Autodesk Fusion 360 part; units mm, degrees
sketch "Sketch1" plane through (0, 0, 0) normal (0, 0, 1) x (1, 0, 0)
  circle A0 centre (0, 0) radius 18.25
  circle A1 centre (0, 0) radius 24.5
  circle A2 centre (0, 0) radius 17.75
  circle A3 centre (0, 0) radius 16.25
  dimension "d1" = 36.5
  dimension "d2" = 49
  dimension "d7" = 35.5
  dimension "d27" = 32.5
extrude "Extrude1" add sketch "Sketch1" along normal blind 15 contours A0 | A1 | A2
extrude "Extrude6" cut sketch "Sketch1" along normal blind 8 contours A2
extrude "Extrude2" cut sketch "Sketch1" along normal blind 6 contours A0
sketch "Sketch5" plane through (0, 0, 0) normal (0, 0, 1) x (1, 0, 0)
  line L0 (-8, 21.5) -> (8, 21.5)
  line L1 (8, 21.5) -> (8, 19.8006)
  line L2 (8, -21.5) -> (-8, -21.5)
  line L3 (-8, 19.8006) -> (-8, 21.5)
  line L4 (-8, 21.5) -> (8, -21.5) construction
  line L5 (8, 21.5) -> (-8, -21.5) construction
  circle A0 centre (0, 0) radius 18.25
  arc A1 (-10.5361, 14.9015) -> (10.5361, 14.9015) centre (0, 0) ccw
  arc A2 (8, 19.8006) -> (10.5361, 14.9015) centre (14, 19.8006) ccw
  arc A3 (-10.5361, 14.9015) -> (-8, 19.8006) centre (-14, 19.8006) ccw
  dimension "d31" = 16
  dimension "d32" = 43
  dimension "d33" = 6
  dimension "d34" = 6
extrude "Extrude7" cut sketch "Sketch5" along normal blind 6 contours L0 L1 L3 A0 A2 A3
chamfer "Chamfer3" distance 7 angle 45 1 edges at (-15.1503, 5.8763, 15)
move_face "OffsetFaces1" offset -1 1 faces at (0, -22.371, 0)
Could you check a few things on this model? Use its own coordinates, in mm. A direction names the side the tool comes from. Give positions to 0.01 mm unless a question says otherwise; leave off trailing zeros. Write each loop counter-clockwise with the first axis right and the second up, starting at its lowest first coordinate (ties: lowest second). Pieces come first, ordered by that corner, then holes. Notation, with made-up numbers: (65.5, 89) -> (110.5, 89) arc R17 ccw to (110.5, 113) -> close; hole circle Ø8 at (2, 12). An arc over 180 degrees is marked (long way). Write each question's results on one line, items separated by ' | '. Start each with the question number.
Q1. We'd pull the mould along X, two halves only. Please class faces 1 (the face through (13.17, -20.66, 7.9)), 2 (the face through (8, 21, 3)), 3 (the face through (9, -22, 15)): +X half, -X half, draft (parallel to the pull), parting line (faces both ways), or undercut.
Q2. Which directions (+Z, -Z, +X, -X, +Y, -Y) give clear straight access to the entire face, cutting with the end or side of a thin tool? Please do faces 4 (the face through (-8.653, 17.078, 3.465)), 5 (the face through (-6, -18, 1)).
Q3. I'm going to push flat-ended pins straight in: pin 1 Ø0.5 at (y, z) = (20.5, 4.5) entering from -X; pin 2 Ø10 at (x, y) = (-8, 1.5) entering from +Z; pin 3 Ø2 at (x, z) = (13.5, 5) entering from -Y; pin 4 Ø3 at (y, z) = (-10, 6.5) entering from +X. Where does each tip first touch, or does it pass through?
Q4. Suppose I cut it at C-C, the plane z = 3.25. List the corners of the cut face in (x, y) for me.
Q5. Suppose I cut it at D-D, the plane z = 7. List the corners of the cut face in (x, y) for me.
Q6. I need wall thicknesses on probe 1 along X at (y, z) = (0, 4.75); probe 2 along X at (y, z) = (0, 7.3). Which ranges of each line are inside material? Lowest first, please.
Outcome:
1) face 1: parting line | face 2: undercut | face 3: draft
2) face 4: -Z | face 5: -Z, +X, -X, +Y, -Y
3) pin 1: x = -13.79 | pin 2: through | pin 3: y = -21.07 | pin 4: x = 22.98
4) outline: circle Ø49 at (0, 0); hole (-10.54, 14.9) arc R18.25 ccw (long way) to (10.54, 14.9) arc R6 cw to (8, 19.8) -> (8, 21.5) -> (-8, 21.5) -> (-8, 19.8) arc R6 cw to start
5) outline: circle Ø49 at (0, 0); hole circle Ø35.5 at (0, 0)
6) probe 1: -24.5 to -18.25, 18.25 to 24.5 | probe 2: -24.5 to -17.75, 17.75 to 24.5
